The listing builds one solid part. Answer for the finished solid, in the listing's coordinates (mm). A direction names the side the tool comes from. Give positions to 0.01 mm unless a question says otherwise; leave off trailing zeros. Write each loop counter-clockwise with the first axis right and the second up, starting at its lowest first coordinate (ties: lowest second). Pieces come first, ordered by that corner, then holes. Notation, with made-up numbers: M 33.25,53.5 L 45.25,53.5 A13 cw 45.25,68.5 Z; hole C 43.25,-40 d2. An arc over 180 degrees is marked long. Answer as a JSON object with one key per item and string values.
```python
from build123d import *

# Parameters (mm, degrees)
F0_W      = 177.8
F0_H      = 44.45
F1_DEPTH  = 31.75
F2_W      = 1.5875
F2_H      = 44.45
F3_DEPTH  = 3.175
F4_W      = 79.85125
F4_H      = 29.21
F5_DEPTH  = 31.751
F7_DEPTH  = 44.451
F8_R      = 5.08
F10_DEPTH = 44.451


with BuildPart() as f1:
    # F0 (on Top) → F1 (new body)
    with BuildSketch(Plane.XY):
        with Locations((-88.9, -22.225)):
            Rectangle(F0_W, F0_H)
    extrude(amount=F1_DEPTH)

    # F2 (on face) → F3 (cut)
    with BuildSketch(Plane(origin=(0, 0, 0), x_dir=(1, 0, 0), z_dir=(0, 0, -1))):
        with Locations((-23.01875, 22.225)):
            Rectangle(F2_W, F2_H)
        with Locations((-134.9375, 22.225)):
            Rectangle(F2_W, F2_H)
    extrude(amount=-F3_DEPTH, mode=Mode.SUBTRACT)

    # F4 (on face) → F5 (cut, through all)
    with BuildSketch(Plane.XY.offset(31.75)):
        with Locations((-86.598125, -22.225)):
            Rectangle(F4_W, F4_H)
    extrude(amount=-F5_DEPTH, mode=Mode.SUBTRACT)

    # F6 (on face) → F7 (cut, through all)
    with BuildSketch(Plane.XZ.offset(44.45)):
        Polygon((-177.8, 31.75), (-177.8, 4.466168), (0, 31.75), align=None)
    extrude(amount=-F7_DEPTH, mode=Mode.SUBTRACT)

    # F8
    f8_edges = [f1.edges().sort_by_distance(p)[0] for p in [
        (-126.52375, -7.62, 6.167315),
        (-46.6725, -7.62, 12.293997),
        (-126.52375, -36.83, 6.167315),
        (-46.6725, -36.83, 12.293997),
    ]]
    fillet(f8_edges, radius=F8_R)

    # F9 (on face) → F10 (cut, through all)
    with BuildSketch(Plane.XZ.offset(44.45)):
        with BuildLine():
            Line((-48.720182, 16.564578), (-90.55252, 10.145306))
            ThreePointArc((-90.55252, 10.145306), (-91.626212, 8.793405), (-90.35989, 7.62))
            Line((-90.35989, 7.62), (-48.4505, 7.62))
            ThreePointArc((-48.4505, 7.62), (-47.193264, 8.140764), (-46.6725, 9.398))
            Line((-46.6725, 9.398), (-46.6725, 14.807149))
            ThreePointArc((-46.6725, 14.807149), (-47.29253, 16.156367), (-48.720182, 16.564578))
        make_face()
    extrude(amount=-F10_DEPTH, mode=Mode.SUBTRACT)


solid = f1.part
```
1. A cutting plane is placed at C-C, the plane x = -42. Give the vertices of the cut face in (y, z) (3 decimals), plus the area to 3 significant figures.
Verdict:
{"outline": "M -44.45,0 L 0,0 L 0,25.305 L -44.45,25.305 Z", "area": "1,120 mm2"}
2. The mould has two halves that part along X. Classify faces 5 (the flat face through (-134.144, -22, 2)), 6 (the flat face through (-70, 0, 16)), 7 (the flat face through (-90.145, -37.353, 17.917)): released by +X, released by -X, zero draft, split by the parting line, or undercut.
Verdict:
{"face 5": "undercut", "face 6": "zero draft", "face 7": "released by -X"}
3. A cutting plane is placed at B-B, the plane x = -77. Give the vertices of the cut face in (y, z), plus the area to 3 significant figures.
Verdict:
{"outline": "M -44.45,0 L -36.83,0 L -36.83,7.62 L -44.45,7.62 Z; M -44.45,12.22 L -36.83,12.22 L -36.83,19.93 L -44.45,19.93 Z; M -7.62,0 L 0,0 L 0,7.62 L -7.62,7.62 Z; M -7.62,12.22 L 0,12.22 L 0,19.93 L -7.62,19.93 Z", "area": "234 mm2"}
4. A cutting plane is placed at D-D, the plane z = 27.5. Give the vertices of the cut face in (x, y).
Verdict:
{"outline": "M -27.7,-44.45 L 0,-44.45 L 0,0 L -27.7,0 Z"}
5. For faces 1 (the cylindrical face through (-48.12, -35.3, 3.59)), 2 (the flat face through (-69.34, -4.37, 13.4)), 3 (the cylindrical face through (-48.2, -9.07, 20.72)), 4 (the flat face through (-23.812, -22, 2)), determine the directions among +Z, -Z, +X, -X, +Y, -Y from which every point of the face is accessible in a straight line to the end or side of a thin tool.
Verdict:
{"face 1": "+Z, -Z", "face 2": "+Y, -Y", "face 3": "+Z, -Z, -X", "face 4": "-Z, +Y, -Y"}
6. Consider line 1 along Y through (x, z) = (-92, 12); line 2 along X through (y, z) = (-31, 22); line 3 along Y through (x, z) = (-48, 23). Determine where each line is inside the solid, lowest interval first.
Verdict:
{"line 1": "y = -44.45 to -36.83, -7.62 to 0", "line 2": "x = -46.67 to 0", "line 3": "y = -44.45 to -35.17, -9.28 to 0"}
7. Flat-ended cylindrical pins translate along their axes: pin 1 (2.5 mm diameter, centred on x = -68, y = -40.5, fed in from +Z); pin 2 (3 mm diameter, centred on x = -46, y = -21.5, fed in from +Z); pin 3 (5 mm diameter, centred on y = -16, z = 17.5, fed in from -X). Find the tip coordinate at first contact, or state that the pin passes through.
Verdict:
{"pin 1": "stops at z = 21.51", "pin 2": "stops at z = 24.92", "pin 3": "stops at x = -46.67"}
